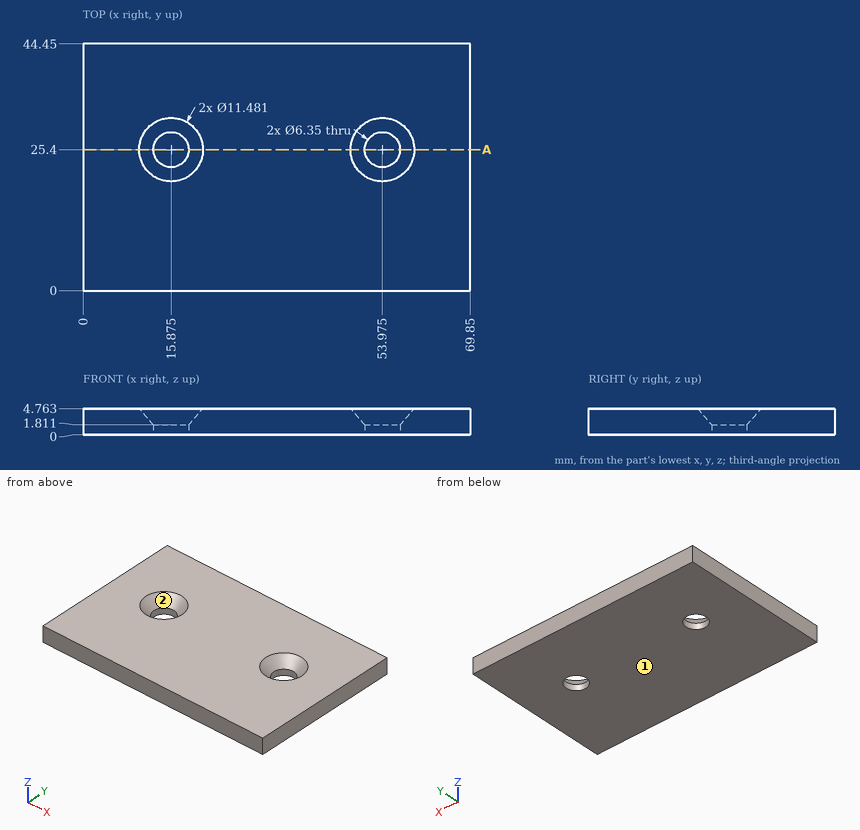
Here's the drawing with two shaded views (mm, measured from the low corner). I have some questions. Coordinates: 2 decimals unless noted, no trailing zeros.
Q1. Will these pins go through, and if not, where does the flat tip stop? pin 1 (7.5 mm diameter, centred on x = 15.875, y = 25.4, fed in from -Z); pin 2 (5.5 mm diameter, centred on x = 53.975, y = 25.4, fed in from -Z).
Q2. Please list where these lines run through material, in increasing order: L1, parallel to X at y = 25.4, z = 1.25; L2, parallel to X at y = 27.5, z = 3.4; L3, parallel to Z at x = 21, y = 23.5 (1 decimal).
Q3. Suppose I cut it at A-A on y = 25.4. Give the number of separate pieces and of enclosed holes in the cut face, and give its area (3 significant figures).
Q4. Thinking about a two-plate mould opening in Y: for the marked faces 1 and 2, which applies, released by +Y, released by -Y, zero draft, split by the parting line, or undercut?
Answer:
1. pin 1: stops at z = 0
1. pin 2: passes through
2. L1: x = 0 to 12.7, 19.05 to 50.8, 57.15 to 69.85
2. L2: x = 0 to 11.83, 19.92 to 49.93, 58.02 to 69.85
2. L3: z = 0 to 4.4
3. separate pieces: 3
3. enclosed holes: 0
3. area: 257 mm2
4. face 1: zero draft
4. face 2: undercut
